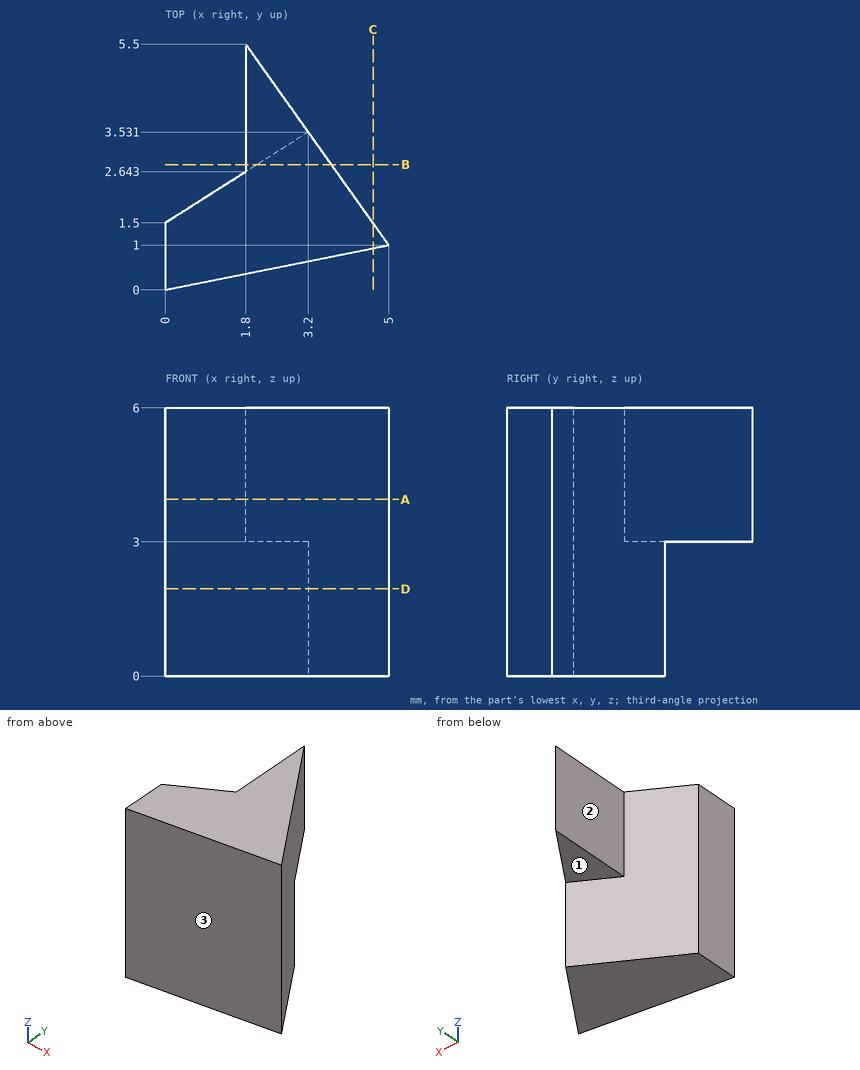
Drawing for the job (mm, zero at the part's lowest x, y, z). A direction names the side the tool comes from. Give positions to 0.01 mm unless a question says otherwise; leave off trailing zeros. Write each loop counter-clockwise with the first axis right and the second up, starting at its lowest first coordinate (ties: lowest second). Pieces come first, ordered by that corner, then holes. Notation, with made-up numbers: M 21,-21 L 72,-21 A9 cw 72,-12 Z; hole C 64.25,-36 d1. An arc over 180 degrees is marked long. Use CSV: the item, a comma, the result in double quotes.
Item 1: Pin check, flat tips, straight feed: P1, Ø3, axis at y = 4, z = 5, coming from the -X side (1 decimal); P2, Ø2, axis at y = 4.5, z = 3, coming from the -X side. Stop position of each tip, or through.
Taken from the geometry:
P1,"stops at x = 1.6"
P2,"stops at x = 1.8"
Item 2: Which spindle directions (+Z, -Z, +X, -X, +Y, -Y) get a long thin tool onto all of the face, cutting with end or side? Do the marked faces 1, 2 and 3. Say none if no direction does.
Taken from the geometry:
face 1,"-Z, -X, +Y"
face 2,"+Z, -Z, -X, +Y"
face 3,"+Z, -Z, +X, -Y"
Item 3: Slice it at D-D on z = 1.95. Write the cut outline in (x, y).
Taken from the geometry:
outline,"M 0,0 L 5,1 L 3.2,3.53 L 0,1.5 Z"
Item 4: Slice it at B-B on y = 2.8. Write the cut outline in (x, z).
Taken from the geometry:
outline,"M 1.8,3 L 2.05,3 L 2.05,0 L 3.72,0 L 3.72,6 L 1.8,6 Z"
Item 5: Drill centre lines: probe 1 along Z at (x, y) = (2.05, 4.2); probe 2 along Y at (x, z) = (3, 3.2) (1 decimal); probe 3 along X at (y, z) = (2.1, 5.5) (1 decimal). Where is each one in solid material? Low to high.
Taken from the geometry:
probe 1,"z = 3 to 6"
probe 2,"y = 0.6 to 3.8"
probe 3,"x = 0.9 to 4.2"
Item 6: Slice it at A-A on z = 3.95. Write the cut outline in (x, y).
Taken from the geometry:
outline,"M 0,0 L 5,1 L 1.8,5.5 L 1.8,2.64 L 0,1.5 Z"
Item 7: Slice it at C-C on x = 4.65. Write the cut outline in (y, z).
Taken from the geometry:
outline,"M 0.93,0 L 1.49,0 L 1.49,6 L 0.93,6 Z"
